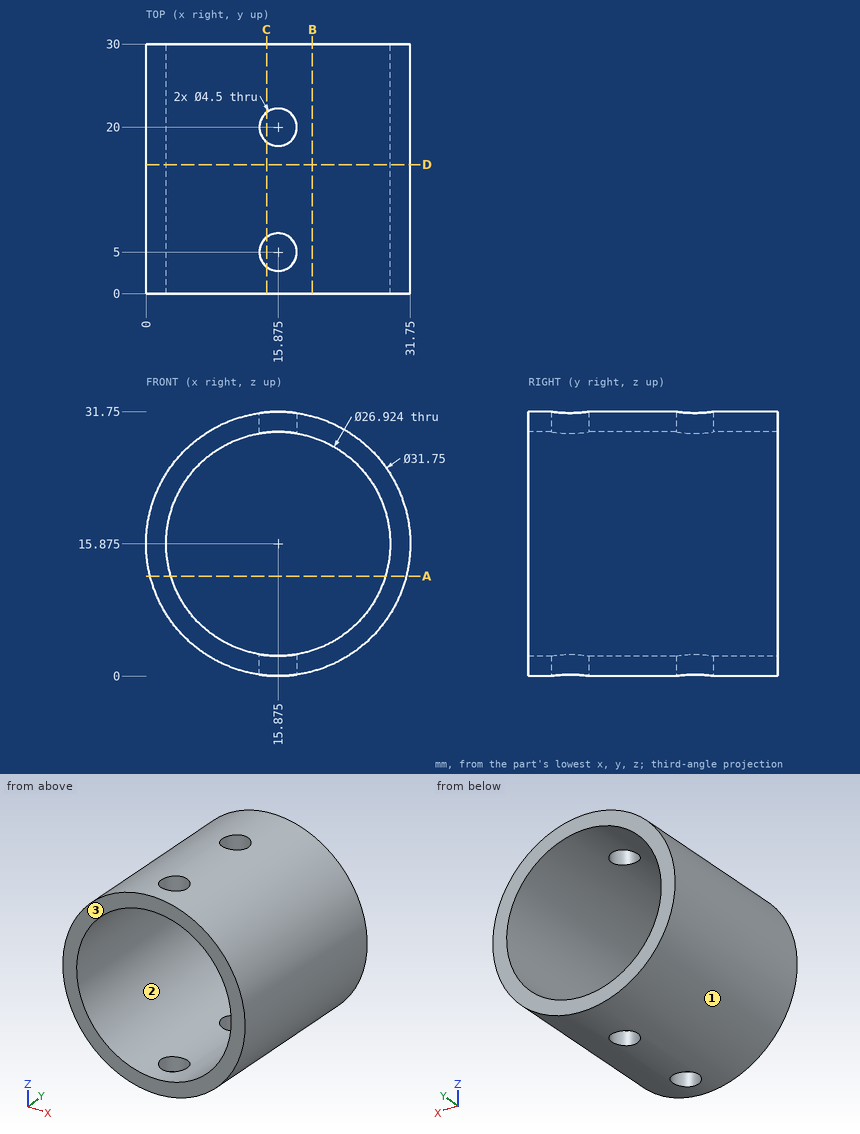
Could you check a few things on this drawing? It's one solid part, dimensions in mm from its lowest x, y, z. Give positions to 0.01 mm unless a question says otherwise; leave off trailing zeros. Loops run counter-clockwise (first coordinate to the right, second up) from the corner with the lowest first, then second, coordinate; pieces in that order, holes last. Notation, with made-up numbers: (-33, 6) -> (-6, 6) arc R16 cw to (-6, 13) -> close; hole circle Ø1 at (87.25, 13.5). An arc over 180 degrees is marked (long way). Use one line per item in the form item = value. Start each with the question number.
1) Imagine slicing it at C-C (x = 14.5). Please give me the cut outline in (y, z).
2) For P1, Ø6, axis at x = 15.875, y = 5, coming from the -Z side; P2, Ø1.5, axis at x = 27, z = 14, coming from the -Y side; P3, Ø12, axis at y = 4, z = 24.5, coming from the +X side; P4, Ø5, axis at y = 13, z = 22.5, coming from the +X side, each with a flat end and sliding along its axis, tell me the tip position at first contact or that it passes through.
3) Imagine slicing it at B-B (x = 20). Please give me the cut outline in (y, z).
4) Imagine slicing it at A-A (z = 12). Please give me the cut outline in (x, y).
5) Thinking about a two-plate mould opening in X: for the marked faces 1, 2 and 3, which applies, +X half, -X half, draft (parallel to the pull), parting line (faces both ways), or undercut?
6) Please list where these lines run through material, in increasing order: line 1 along X through (y, z) = (16, 5.5); line 2 along Z through (x, y) = (12.5, 18); line 3 along Z through (x, y) = (11.5, 5).
7) Imagine slicing it at D-D (y = 15.5). Please give me the cut outline in (x, z) (3 decimals).
Check values:
q1.outline = (0, 0.06) -> (3.22, 0.06) -> (3.22, 2.48) -> (0, 2.48) -> close; (0, 29.27) -> (3.22, 29.27) -> (3.22, 31.69) -> (0, 31.69) -> close; (6.78, 0.06) -> (18.22, 0.06) -> (18.22, 2.48) -> (6.78, 2.48) -> close; (6.78, 29.27) -> (18.22, 29.27) -> (18.22, 31.69) -> (6.78, 31.69) -> close; (21.78, 0.06) -> (30, 0.06) -> (30, 2.48) -> (21.78, 2.48) -> close; (21.78, 29.27) -> (30, 29.27) -> (30, 31.69) -> (21.78, 31.69) -> close
q2.P1 = 0
q2.P2 = through
q2.P3 = 31.53
q2.P4 = 31.2
q3.outline = (0, 0.55) -> (30, 0.55) -> (30, 3.06) -> (0, 3.06) -> close; (0, 28.69) -> (30, 28.69) -> (30, 31.2) -> (0, 31.2) -> close
q4.outline = (0.48, 0) -> (2.98, 0) -> (2.98, 30) -> (0.48, 30) -> close; (28.77, 0) -> (31.27, 0) -> (31.27, 30) -> (28.77, 30) -> close
q5.face_1 = parting line
q5.face_2 = undercut
q5.face_3 = draft
q6.line_1 = 3.86 to 7.3, 24.45 to 27.89
q6.line_2 = 0.36 to 2.84, 28.91 to 31.39
q6.line_3 = 0.61 to 3.14, 28.61 to 31.14
q7.outline = circle Ø31.75 at (15.875, 15.875); hole circle Ø26.924 at (15.875, 15.875)
